Can you work these out from the model? Positions are in its coordinate system, mm. A direction names the side the tool comes from. Coordinates: 2 decimals unless noted, no trailing zeros. Order: outer loops, then holes, each group sorted by start corner. A loop starts at its lowest first (then second) coordinate and runs counter-clockwise, first axis right, second up. Notation, with made-up numbers: (21.5, -9) -> (28.5, -9) arc R21 ccw to (28.5, -1) -> close; hole circle Ø8 at (54, -29). An arc over 180 degrees is marked (long way). Answer as CSV lines item,"result".
from build123d import *

# Parameters (mm, degrees)
BOSS_EXTRUDE1_DEPTH = 13
BOSS_EXTRUDE2_DEPTH = 5
FILLET1_R           = 2
SKETCH3_R           = 0.75
CUT_EXTRUDE1_DEPTH  = 4.9
SKETCH4_R           = 2.25
BOSS_EXTRUDE3_DEPTH = 3


with BuildPart() as part:
    # Sketch1 → Boss-Extrude1 (new body)
    with BuildSketch(Plane(origin=(0, 0, 0), x_dir=(1, 0, 0), z_dir=(0, 1, 0))):
        Polygon((0, 20.5), (5, 22), (11.5, 22), (23, 22), (23, 18.7), (27.4, 18.7), (27.4, 16.2), (23, 16.2), (23, 0), (0, 0), (0, 16.2), (-4.4, 16.2), (-4.4, 18.7), (0, 18.7), align=None)
    extrude(amount=BOSS_EXTRUDE1_DEPTH)

    # Sketch2 → Boss-Extrude2 (add)
    with BuildSketch(Plane(origin=(0, 0, -22), x_dir=(-1, 0, 0), z_dir=(0, 0, -1))):
        with BuildLine():
            Line((-23, 9.994281042), (-23, 3.005718958))
            ThreePointArc((-23, 3.005718958), (-17.997144773, 0.400000668), (-12.996731055, 3.010401189))
            ThreePointArc((-12.996731055, 3.010401189), (-12.16968389, 3.737727457), (-11.1, 4))
            ThreePointArc((-11.1, 4), (-8.6, 6.5), (-11.1, 9))
            ThreePointArc((-11.1, 9), (-12.16968389, 9.262272543), (-12.996731055, 9.989598811))
            ThreePointArc((-12.996731055, 9.989598811), (-17.997144773, 12.599999332), (-23, 9.994281042))
        make_face()
    extrude(amount=BOSS_EXTRUDE2_DEPTH)

    # Fillet1
    fillet1_edges = [part.edges().sort_by_distance(p)[0] for p in [
        (-4.4, 0, -17.45),
        (27.4, 13, -17.45),
        (27.4, 0, -17.45),
        (-4.4, 13, -17.45),
    ]]
    fillet(fillet1_edges, radius=FILLET1_R)

    # Sketch3 → Cut-Extrude1 (cut)
    with BuildSketch(Plane(origin=(0, 0, -18.7), x_dir=(-1, 0, 0), z_dir=(0, 0, -1))):
        with Locations((-25.65, 6.5)):
            Circle(SKETCH3_R)
        with Locations((-24, 10.25)):
            Circle(SKETCH3_R)
        with Locations((-24, 2.75)):
            Circle(SKETCH3_R)
        with Locations((1, 2.75)):
            Circle(SKETCH3_R)
        with Locations((2.65, 6.5)):
            Circle(SKETCH3_R)
        with Locations((1, 10.25)):
            Circle(SKETCH3_R)
    extrude(amount=-CUT_EXTRUDE1_DEPTH, mode=Mode.SUBTRACT)

    # Sketch4 → Boss-Extrude3 (add)
    with BuildSketch(Plane(origin=(0, 0, -27), x_dir=(-1, 0, 0), z_dir=(0, 0, -1))):
        with Locations((-18, 6.5)):
            Circle(SKETCH4_R)
    extrude(amount=BOSS_EXTRUDE3_DEPTH)


solid = part.part
Q1. If I drill on line 1 (Y direction, x = -1, z = -17.15); line 2 (Z direction, x = 14.5, y = 1); line 3 (X direction, y = 5, z = -10.5), over which ranges is the centre line in solid material (lowest first)?
Solution:
line 1,"0 to 2, 3.5 to 9.5, 11 to 13"
line 2,"-22 to 0"
line 3,"0 to 23"
Q2. Imagine slicing it at B-B (x = 24). List the corners of the cut face in (y, z) for me.
Solution:
outline,"(0, -18.7) -> (2, -18.7) -> (2, -16.2) -> (0, -16.2) -> close; (3.5, -18.7) -> (9.5, -18.7) -> (9.5, -16.2) -> (3.5, -16.2) -> close; (11, -18.7) -> (13, -18.7) -> (13, -16.2) -> (11, -16.2) -> close"
Q3. We'd pull the mould along Y, two halves only. Please class faces 1 (the cylindrical face through (-0.25, 2.78, -17.47)), 2 (the flat face through (16, 5, -27)), 3 (the cylindrical face through (26.8, 12.43, -17.43)), 4 (the cylindrical face through (15.854, 7.176, -28.479)): pulls with the +Y half, pulls with the -Y half, needs draft (parallel to the pull), parting line crosses it, or undercut.
Solution:
face 1,"undercut"
face 2,"needs draft"
face 3,"pulls with the +Y half"
face 4,"parting line crosses it"
Q4. Imagine slicing it at A-A (y = 6.5). List the corners of the cut face in (x, z) for me, and give its area (3 significant figures).
Solution:
outline,"(-4.4, -18.7) -> (-3.4, -18.7) -> (-3.4, -16.2) -> (-4.4, -16.2) -> close; (-1.9, -18.7) -> (0, -18.7) -> (0, -20.5) -> (5, -22) -> (8.6, -22) -> (8.6, -27) -> (15.75, -27) -> (15.75, -30) -> (20.25, -30) -> (20.25, -27) -> (23, -27) -> (23, -18.7) -> (24.9, -18.7) -> (24.9, -16.2) -> (23, -16.2) -> (23, 0) -> (0, 0) -> (0, -16.2) -> (-1.9, -16.2) -> close; (26.4, -18.7) -> (27.4, -18.7) -> (27.4, -16.2) -> (26.4, -16.2) -> close"
area,"602 mm2"
Q5. Imagine slicing it at C-C (z = -17). List the corners of the cut face in (x, y) for me, and give its area (3 significant figures).
Solution:
outline,"(-4.4, 2) arc R2 ccw to (-2.4, 0) -> (25.4, 0) arc R2 ccw to (27.4, 2) -> (27.4, 11) arc R2 ccw to (25.4, 13) -> (-2.4, 13) arc R2 ccw to (-4.4, 11) -> close; hole circle Ø1.5 at (-2.65, 6.5); hole circle Ø1.5 at (-1, 2.75); hole circle Ø1.5 at (-1, 10.25); hole circle Ø1.5 at (24, 2.75); hole circle Ø1.5 at (24, 10.25); hole circle Ø1.5 at (25.65, 6.5)"
area,"399 mm2"
Q6. Which directions (+Z, -Z, +X, -X, +Y, -Y) give clear straight access to the entire face, cutting with the end or side of a thin tool? Please do faces 5 (the cylindrical face through (17.9, 12.6, -24.5)), 6 (the cylindrical face through (8.6, 6.4, -24.5)), 7 (the flat face through (0, 6, -20)), 8 (the flat face through (24.7, 6.4, -16.2)), 9 (the cylindrical face through (12.156, 9.255, -24.465)).
Solution:
face 5,"-Z, +Y"
face 6,"-Z, -X"
face 7,"-Z, -X, +Y, -Y"
face 8,"+Z, +X, +Y, -Y"
face 9,"-Z, -X, +Y"
Q7. For P1, Ø1, axis at x = 7, y = 10.5, coming from the -Z side; P2, Ø4, axis at y = 9.5, z = -11, coming from the -X side; P3, Ø3.5, axis at x = -1.5, y = 9, coming from the -Z side (3 decimals), each with a flat end and sliding along its axis, tell me the tip position at first contact or that it passes through.
Solution:
P1,"z = -22"
P2,"x = 0"
P3,"z = -20.575"
Q8. Imagine slicing it at D-D (x = 18.5). List the corners of the cut face in (y, z) for me.
Solution:
outline,"(0, -22) -> (0.42, -22) -> (0.42, -27) -> (4.31, -27) -> (4.31, -30) -> (8.69, -30) -> (8.69, -27) -> (12.58, -27) -> (12.58, -22) -> (13, -22) -> (13, 0) -> (0, 0) -> close"
